Can you work these out from the drawing? Everything is in mm from the part's minimum corner. A direction names the side the tool comes from. Round coordinates to 2 decimals unless told otherwise and drop trailing zeros. Loops run counter-clockwise (first coordinate to the right, second up) from the corner with the lowest first, then second, coordinate; pieces in that order, holes last. Notation, with made-up numbers: M -15.75,46 L 16.25,46 A23 ccw 16.25,59 Z; hole C 12,-1 d2. An arc over 180 degrees is marked long. Use a Markdown table: item, result.
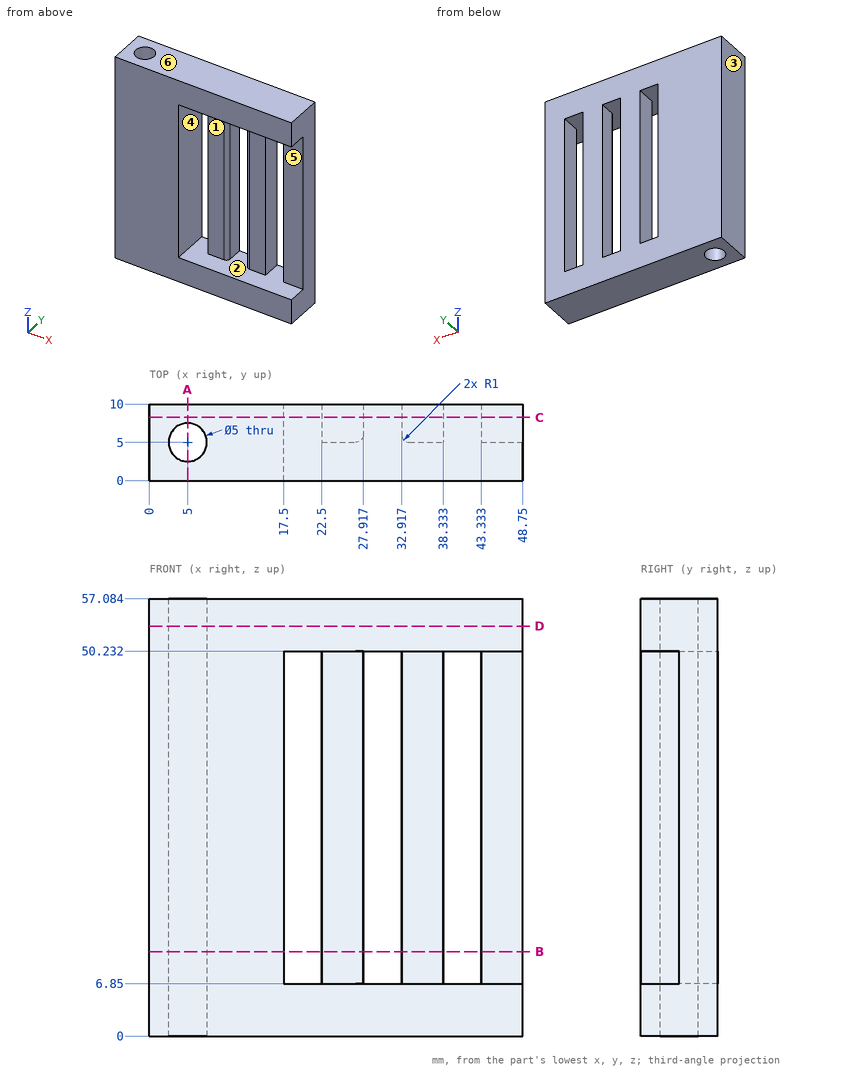
1. Which directions (+Z, -Z, +X, -X, +Y, -Y) give clear straight access to the entire face, cutting with the end or side of a thin tool? Please do the marked faces 4, 5 and 6.
Answer sheet:
| item | result |
|---|---|
| face 4 | +Y, -Y |
| face 5 | +X, -Y |
| face 6 | +Z, +X, -X, +Y, -Y |
2. We'd pull the mould along X, two halves only. Please class the marked faces 1, 2 and 3: +X half, -X half, draft (parallel to the pull), parting line (faces both ways), or undercut.
Answer sheet:
| item | result |
|---|---|
| face 1 | draft |
| face 2 | undercut |
| face 3 | -X half |
3. Imagine slicing it at B-B, the plane z = 11. Write out the boundary of the cut face in (x, y), then the cut area to 3 significant figures.
Answer sheet:
| item | result |
|---|---|
| outline | M 0,0 L 17.5,0 L 17.5,10 L 0,10 Z; M 22.5,5 L 26.92,5 A1 ccw 27.92,6 L 27.92,10 L 22.5,10 Z; M 32.92,6 A1 ccw 33.92,5 L 38.33,5 L 38.33,10 L 32.92,10 Z; M 43.33,5 L 48.75,5 L 48.75,10 L 43.33,10 Z; hole C 5,5 d5 |
| area | 236 mm2 |
4. Imagine slicing it at C-C, the plane y = 8.25. Write out the boundary of the cut face in (x, z).
Answer sheet:
| item | result |
|---|---|
| outline | M 0,0 L 48.75,0 L 48.75,57.08 L 0,57.08 Z; hole M 17.5,6.85 L 22.5,6.85 L 22.5,50.23 L 17.5,50.23 Z; hole M 27.92,6.85 L 32.92,6.85 L 32.92,50.23 L 27.92,50.23 Z; hole M 38.33,6.85 L 43.33,6.85 L 43.33,50.23 L 38.33,50.23 Z |
5. Imagine slicing it at A-A, the plane x = 5. Write out the boundary of the cut face in (y, z).
Answer sheet:
| item | result |
|---|---|
| outline | M 0,0 L 2.5,0 L 2.5,57.08 L 0,57.08 Z; M 7.5,0 L 10,0 L 10,57.08 L 7.5,57.08 Z |
6. I need wall thicknesses on probe 1 along X at (y, z) = (8.5, 37); probe 2 along Y at (x, z) = (5, 27); probe 3 along Z at (x, y) = (38.5, 6). Which ranges of each line are inside material? Lowest first, please. Write a range as from..to.
Answer sheet:
| item | result |
|---|---|
| probe 1 | 0..17.5, 22.5..27.92, 32.92..38.33, 43.33..48.75 |
| probe 2 | 0..2.5, 7.5..10 |
| probe 3 | 0..6.85, 50.23..57.08 |
7. For pin 1 Ø2.5 at (x, z) = (45, 18.5) entering from -Y; pin 2 Ø4 at (x, y) = (5, 5) entering from +Z, each with a flat end and sliding along its axis, tell me the tip position at first contact or that it passes through.
Answer sheet:
| item | result |
|---|---|
| pin 1 | y = 5 |
| pin 2 | through |
8. Imagine slicing it at D-D, the plane z = 53.5. Write out the boundary of the cut face in (x, y).
Answer sheet:
| item | result |
|---|---|
| outline | M 0,0 L 48.75,0 L 48.75,10 L 0,10 Z; hole C 5,5 d5 |
